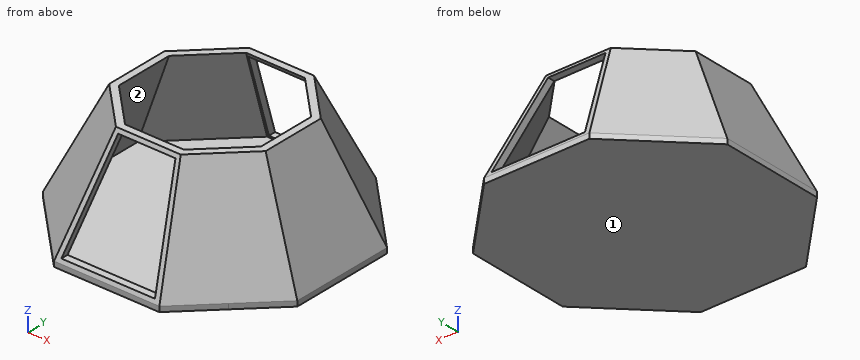
from build123d import *

# Parameters (mm, degrees)
F1_DEPTH = 2
F6_T     = -2.5
F8_DEPTH = 84.8


with BuildPart() as f1:
    # F0 (on Top) → F1 (new body)
    with BuildSketch(Plane.XY):
        with BuildLine():
            ThreePointArc((34.4714555828, -34.4714555828), (45.0391272099, -18.6558173278), (48.75, 0))
            ThreePointArc((48.75, 0), (45.0391271917, 18.6558173718), (34.4714555154, 34.4714556502))
            ThreePointArc((34.4714555154, 34.4714556502), (18.655817355, 45.0391271987), (1.543e-07, 48.75))
            ThreePointArc((1.543e-07, 48.75), (-18.6558172398, 45.0391272464), (-34.4714555572, 34.4714556085))
            ThreePointArc((-34.4714555572, 34.4714556085), (-45.039127203, 18.6558173446), (-48.75, 0))
            ThreePointArc((-48.75, 0), (-45.0391272099, -18.6558173278), (-34.4714555828, -34.4714555828))
            ThreePointArc((-34.4714555828, -34.4714555828), (-18.6558173238, -45.0391272116), (8.6e-09, -48.75))
            ThreePointArc((8.6e-09, -48.75), (18.6558173318, -45.0391272083), (34.4714555828, -34.4714555828))
        make_face()
        with BuildLine():
            Line((48.75, -20.1929111657), (48.75, 0))
            ThreePointArc((48.75, 0), (45.0391272099, -18.6558173278), (34.4714555828, -34.4714555828))
            Line((34.4714555828, -34.4714555828), (48.75, -20.1929111657))
        make_face()
        with BuildLine():
            ThreePointArc((34.4714555154, 34.4714556502), (45.0391271917, 18.6558173718), (48.75, 0))
            Line((48.75, 0), (48.75, 20.1929111657))
            Line((48.75, 20.1929111657), (34.4714555154, 34.4714556502))
        make_face()
        with BuildLine():
            ThreePointArc((1.543e-07, 48.75), (18.655817355, 45.0391271987), (34.4714555154, 34.4714556502))
            Line((34.4714555154, 34.4714556502), (20.1929111657, 48.75))
            Line((20.1929111657, 48.75), (1.543e-07, 48.75))
        make_face()
        with BuildLine():
            Line((20.1929111657, -48.75), (34.4714555828, -34.4714555828))
            ThreePointArc((34.4714555828, -34.4714555828), (18.6558173318, -45.0391272083), (8.6e-09, -48.75))
            Line((8.6e-09, -48.75), (20.1929111657, -48.75))
        make_face()
        with BuildLine():
            ThreePointArc((-34.4714555572, 34.4714556085), (-18.6558172398, 45.0391272464), (1.543e-07, 48.75))
            Line((1.543e-07, 48.75), (-20.1929111657, 48.75))
            Line((-20.1929111657, 48.75), (-34.4714555572, 34.4714556085))
        make_face()
        with BuildLine():
            Line((-20.1929111657, -48.75), (8.6e-09, -48.75))
            ThreePointArc((8.6e-09, -48.75), (-18.6558173238, -45.0391272116), (-34.4714555828, -34.4714555828))
            Line((-34.4714555828, -34.4714555828), (-20.1929111657, -48.75))
        make_face()
        with BuildLine():
            ThreePointArc((-48.75, 0), (-45.039127203, 18.6558173446), (-34.4714555572, 34.4714556085))
            Line((-34.4714555572, 34.4714556085), (-48.75, 20.1929111657))
            Line((-48.75, 20.1929111657), (-48.75, 0))
        make_face()
        with BuildLine():
            Line((-48.75, -20.1929111657), (-34.4714555828, -34.4714555828))
            ThreePointArc((-34.4714555828, -34.4714555828), (-45.0391272099, -18.6558173278), (-48.75, 0))
            Line((-48.75, 0), (-48.75, -20.1929111657))
        make_face()
    extrude(amount=F1_DEPTH)

    # F4 (on face) → F5 section 0
    with BuildSketch(Plane.XY.offset(2)):
        Polygon((-48.75, 20.1929111657), (-48.75, -20.1929111657), (-20.1929111657, -48.75), (20.1929111657, -48.75), (48.75, -20.1929111657), (48.75, 20.1929111657), (20.1929111657, 48.75), (-20.1929111657, 48.75), align=None)
    # F3 (on offset) → F5 section 1
    with BuildSketch(Plane.XY.offset(42)):
        Polygon((-30, 12.4264068712), (-30, -12.4264068712), (-12.4264068712, -30), (12.4264068712, -30), (30, -12.4264068712), (30, 12.4264068712), (12.4264068712, 30), (-12.4264068712, 30), align=None)
    loft()

    # F6
    f6_openings = [f1.faces().sort_by_distance(p)[0] for p in [
        (0, 0, 42),
    ]]
    offset(amount=F6_T, openings=f6_openings, kind=Kind.INTERSECTION)

    # F7 (on Front) → F8 (cut, symmetric)
    with BuildSketch(Plane.XZ):
        Polygon((0, 3.399281064), (17.9396793246, 3.399281064), (10.999482125, 40.508095175), (0, 40.508095175), (-10.999482125, 40.508095175), (-17.9396793246, 3.399281064), align=None)
    extrude(amount=F8_DEPTH, both=True, mode=Mode.SUBTRACT)


solid = f1.part
For this review, take the finished solid that the model builds, in its own axes (mm). Face numbers are marked on the shaded views. Round coordinates to 2 decimals unless told otherwise and drop trailing zeros. Use a Markdown table: item, result. Add a question column.
Item 1: To check wall thickness, follow line 1 along X through (y, z) = (7.5, 20.5); line 2 along Z through (x, y) = (-10, 38.5); line 3 along Y through (x, z) = (32.5, 6). State the ranges of each line that lie inside material, in increasing order.
Item 2: Insertion check: pin 1 (0.8 mm diameter, centred on x = 3, y = 47, fed in from +Z); pin 2 (4 mm diameter, centred on y = -19.5, z = 15, fed in from -X); pin 3 (5 mm diameter, centred on y = 18, z = 36, fed in from +X). Each pin has a flat end and moves straight along its axis. Give the tip position at first contact, or say it passes through.
Item 3: Add section A-A, the plane x = 9. State how many separate pieces and enclosed holes the cut face has, then the cut area to 3 significant figures.
Item 4: Mouldability with a two-part tool opening along Y and no side actions: class the marked faces 1 and 2 as released by +Y, released by -Y, zero draft, split by the parting line, or undercut.
Geometry results:
| question | item | result |
|---|---|---|
| 1 | line 1 | x = -40.08 to -37.32, 37.32 to 40.08 |
| 1 | line 2 | z = 0 to 2.5 |
| 1 | line 3 | y = -33.79 to -29.89, 29.89 to 33.79 |
| 2 | pin 1 | stops at z = 3.4 |
| 2 | pin 2 | stops at x = -43.22 |
| 2 | pin 3 | stops at x = 31.4 |
| 3 | separate pieces | 3 |
| 3 | enclosed holes | 0 |
| 3 | area | 257 mm² |
| 4 | face 1 | zero draft |
| 4 | face 2 | undercut |
